Input: part model. Units: mm. Frame: model coordinates. Face numbers are marked on the shaded views. Give positions to 0.01 mm unless a question says otherwise; leave off trailing zeros. Loops run counter-clockwise (first coordinate to the right, second up) from the corner with the lowest first, then second, coordinate; pieces in that order, holes last. Notation, with made-up numbers: (80, 68.5) - (123, 68.5) arc R30 ccw to (123, 90.5) - close; hole circle Ø4 at (53.25, -18). An arc over 180 degrees is marked (long way). One line per item, written item: value.
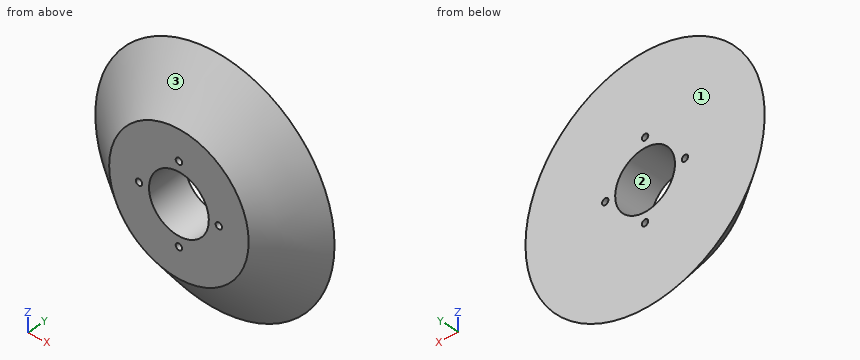
from build123d import *

# Parameters (mm, degrees)
SKETCH_2_R          = 60
SKETCH_1_R          = 35
SKETCH_3_R          = 1.6
SKETCH_3_R_2        = 15
CUT_EXTRUDE_1_DEPTH = 88.177979031


with BuildPart() as part:
    # ｽｹｯﾁ2 → ﾛﾌﾄ1 section 0
    with BuildSketch(Plane(origin=(0, 20, 0), x_dir=(1, 0, 0), z_dir=(0, 1, 0))):
        Circle(SKETCH_2_R)
    # ｽｹｯﾁ1 → ﾛﾌﾄ1 section 1
    with BuildSketch(Plane(origin=(0, 0, 0), x_dir=(1, 0, 0), z_dir=(0, 1, 0))):
        Circle(SKETCH_1_R)
    loft()

    # ｽｹｯﾁ3 → ｶｯﾄ - 押し出し1 (cut, through all)
    with BuildSketch(Plane(origin=(0, 20, 0), x_dir=(1, 0, 0), z_dir=(0, 1, 0))):
        with Locations(Location((0, 20, 0), (0, 0, 270))):
            Circle(SKETCH_3_R)
        with Locations(Location((20, 0, 0), (0, 0, 270))):
            Circle(SKETCH_3_R)
        with Locations(Location((0, -20, 0), (0, 0, 270))):
            Circle(SKETCH_3_R)
        with Locations(Location((-20, 0, 0), (0, 0, 270))):
            Circle(SKETCH_3_R)
        with Locations(Location((0, 0, 0), (0, 0, 270))):
            Circle(SKETCH_3_R_2)
    extrude(amount=-CUT_EXTRUDE_1_DEPTH, mode=Mode.SUBTRACT)


solid = part.part
Item 1: Section B-B, the plane y = 6. Output: boundary loops of the cut face in (x, z).
Verdict:
outline: circle Ø85 at (0, 0); hole circle Ø3.2 at (-20, 0); hole circle Ø30 at (0, 0); hole circle Ø3.2 at (0, -20); hole circle Ø3.2 at (0, 20); hole circle Ø3.2 at (20, 0)
Item 2: Material intervals for L1, parallel to Z at x = -13.5, y = 3.5; L2, parallel to X at y = 14.25, z = 0; L3, parallel to X at y = 6.75, z = -20, sorted ascending.
Verdict:
L1: z = -36.99 to -6.54, 6.54 to 36.99
L2: x = -52.81 to -21.6, -18.4 to -15, 15 to 18.4, 21.6 to 52.81
L3: x = -38.56 to -1.6, 1.6 to 38.56
Item 3: Section A-A, the plane y = 12. Output: boundary loops of the cut face in (x, z), and give its area (3 significant figures).
Verdict:
outline: circle Ø100 at (0, 0); hole circle Ø3.2 at (-20, 0); hole circle Ø30 at (0, 0); hole circle Ø3.2 at (0, -20); hole circle Ø3.2 at (0, 20); hole circle Ø3.2 at (20, 0)
area: 7,110 mm^2
Item 4: Pin query (flat end, axial travel): P1, Ø5, axis at y = 13, z = 31, coming from the +X side; P2, Ø2, axis at y = 9.5, z = 26.5, coming from the -X side; P3, Ø2, axis at x = -43.5, y = 14, coming from the -Z side. Return the tip coordinate at first contact, or that it passes through.
Verdict:
P1: stops at x = 45.04
P2: stops at x = -40.31
P3: stops at z = -31.97
Item 5: Draft query along Z for the marked faces 1, 2 and 3. Return one class per face: pulls with the +Z half, pulls with the -Z half, needs draft (parallel to the pull), parting line crosses it, or undercut.
Verdict:
face 1: needs draft
face 2: undercut
face 3: parting line crosses it
